from build123d import *

# Parameters (mm, degrees)
SKETCH1_R                = 0.635
BOSS_EXTRUDE1_DEPTH      = 127
BOSS_EXTRUDE2_DEPTH      = 0.635
BOSS_EXTRUDE2_DEPTH_BACK = 0.635
FILLET1_R                = 0.508


with BuildPart() as part:
    # Sketch1 → Boss-Extrude1 (new body)
    with BuildSketch(Plane(origin=(0, 0, 0), x_dir=(1, 0, 0), z_dir=(0, 1, 0))):
        Circle(SKETCH1_R)
    extrude(amount=BOSS_EXTRUDE1_DEPTH)

    # Sketch2 → Boss-Extrude2 (add, two sides)
    with BuildSketch(Plane.XY) as boss_extrude2_sk:
        with BuildLine():
            Line((-1.905, 127), (0.635, 127))
            Line((0.635, 127), (0.635, 136.158420865))
            add(Edge.make_bspline(
                [(0.635, 136.158420865), (4.153630903, 141.818791199), (4.114669439, 141.992054971), (4.005734255, 144.307253859)],
                knots=[0, 0, 0, 0, 1, 1, 1, 1], degree=3))
            ThreePointArc((4.005734255, 144.307253859), (-0.739604915, 148.557439765), (-5.289336973, 144.098486718))
            add(Edge.make_bspline(
                [(-1.905, 136.158420865), (-3.718327637, 138.500370735), (-5.598593588, 140.574024695), (-5.289336973, 144.098486718)],
                knots=[0, 0, 0, 0, 1, 1, 1, 1], degree=3))
            Line((-1.905, 136.158420865), (-1.905, 127))
        make_face()
        with BuildLine():
            add(Edge.make_bspline(
                [(-0.297199842, 136.880205631), (-0.107641201, 137.223242161), (0.313462848, 137.90543324), (1.149179042, 139.110045469), (1.915323622, 140.205619235), (2.462394721, 141.272158502), (2.748069771, 142.085078064), (2.871045761, 142.816900596), (2.888508164, 143.458131128), (2.864325917, 143.820492805), (2.844879762, 143.995433072)],
                knots=[0, 0, 0, 0, 0.125, 0.25, 0.5, 0.625, 0.75, 0.875, 0.9375, 1, 1, 1, 1], degree=3))
            Line((-0.297199842, 136.880205631), (-0.972800158, 136.880205631))
            add(Edge.make_bspline(
                [(-0.972800158, 136.880205631), (-1.198644094, 137.171887712), (-1.663408729, 137.76102171), (-2.517671044, 138.87030936), (-3.240026875, 139.952731811), (-3.749328451, 141.06606592), (-4.016349262, 141.942088489), (-4.13205868, 142.739298518), (-4.150496215, 143.42980398), (-4.131124798, 143.810295526), (-4.114879762, 143.995433072)],
                knots=[0, 0, 0, 0, 0.125, 0.25, 0.5, 0.625, 0.75, 0.875, 0.9375, 1, 1, 1, 1], degree=3))
            ThreePointArc((-4.114879762, 143.995433072), (-0.635, 147.191296776), (2.844879762, 143.995433072))
        make_face(mode=Mode.SUBTRACT)
    extrude(amount=BOSS_EXTRUDE2_DEPTH)
    extrude(boss_extrude2_sk.sketch, amount=-BOSS_EXTRUDE2_DEPTH_BACK)

    # Fillet1
    fillet1_edges = [part.edges().sort_by_distance(p)[0] for p in [
        (-0.739604915, 148.557439765, -0.635),
        (0.635, 131.579210433, 0.635),
        (-0.739604915, 148.557439765, 0.635),
        (-1.905, 131.579210433, -0.635),
        (-1.905, 131.579210433, 0.635),
        (0.635, 131.579210433, -0.635),
    ]]
    fillet(fillet1_edges, radius=FILLET1_R)


solid = part.part
Work out the finished part from the listing and answer in its coordinate system (mm). A direction names the side the tool comes from. Round coordinates to 2 decimals unless told otherwise and drop trailing zeros. Loops run counter-clockwise (first coordinate to the right, second up) from the corner with the lowest first, then second, coordinate; pieces in that order, holes last. Notation, with made-up numbers: (65, 78) - (105, 78) arc R21 cw to (105, 86) - close; hole circle Ø9 at (57.5, 63). An arc over 180 degrees is marked (long way). Use one line per item in the form item = value. Start each with the question number.
(1) Find section A-A on y = 51.5. Determine the outline of the cut face in (x, z) (3 decimals).
(2) Which of the six approach directions +Z, -Z, +X, -X, +Y, -Y give full straight-line access (tool end or side, diameter ignored) to faces 1 (the face through (0, 137, -0.635)), 2 (the face through (-0.71, 147.19, 0.01))?
(3) Flat-ended cylindrical pins translate along their axes: P1, Ø0.6, axis at x = -1.5, z = -0.5, coming from the -Y side; P2, Ø4, axis at x = 0.5, y = 16, coming from the +Z side (3 decimals). Find the tip coordinate at first contact, or state that the pin passes through.
(4) Consider line 1 (X direction, y = 100, z = -0.1); line 2 (Y direction, x = -2, z = 0.2); line 3 (Y direction, x = 1.75, z = -0.4). Determine where each line is inside the solid, lowest interval first.
Answer list:
q1.outline = circle Ø1.27 at (0, 0)
q2.face_1 = -Z, +X, -X, +Y, -Y
q2.face_2 = +Z, -Z
q3.P1 = 127
q3.P2 = 0.635
q4.line_1 = -0.63 to 0.63
q4.line_2 = 136.29 to 138.2, 146.91 to 148.35
q4.line_3 = 138.12 to 140, 146.25 to 147.81
